Design review of the part built by this model. Coordinates are the model's own, in mm. A direction names the side the tool comes from. Round coordinates to 2 decimals unless told otherwise and drop trailing zeros. Loops run counter-clockwise (first coordinate to the right, second up) from the corner with the lowest first, then second, coordinate; pieces in that order, holes last. Notation, with made-up numbers: M 77.5,72.5 L 136.5,72.5 A14 cw 136.5,76.5 Z; hole C 24.25,-39 d7. An arc over 180 degrees is marked long. Answer as CSV lines item,"result". Start each with the question number.
from build123d import *

# Parameters (mm, degrees)
SKETCH5_W           = 1600
SKETCH5_H           = 900
BOSS_EXTRUDE4_DEPTH = 100
SKETCH6_R           = 50
BOSS_EXTRUDE5_DEPTH = 700
SKETCH8_R           = 75
CUT_EXTRUDE2_DEPTH  = 90
FILLET2_R           = 80


with BuildPart() as part:
    # Sketch5 → Boss-Extrude4 (new body)
    with BuildSketch(Plane(origin=(0, 0, 0), x_dir=(1, 0, 0), z_dir=(0, 1, 0))):
        Rectangle(SKETCH5_W, SKETCH5_H)
    extrude(amount=BOSS_EXTRUDE4_DEPTH)

    # Sketch6 → Boss-Extrude5 (add)
    with BuildSketch(Plane(origin=(0, 100, 0), x_dir=(1, 0, 0), z_dir=(0, 1, 0))):
        with Locations((-710, 360)):
            Circle(SKETCH6_R)
        with Locations((710, 360)):
            Circle(SKETCH6_R)
        with Locations((710, -360)):
            Circle(SKETCH6_R)
        with Locations((-710, -360)):
            Circle(SKETCH6_R)
    extrude(amount=-BOSS_EXTRUDE5_DEPTH)

    # Sketch8 → Cut-Extrude2 (cut)
    with BuildSketch(Plane(origin=(0, 100, 0), x_dir=(1, 0, 0), z_dir=(0, 1, 0))):
        with Locations((400, 0)):
            Circle(SKETCH8_R)
    cut_extrude2 = extrude(amount=-CUT_EXTRUDE2_DEPTH, mode=Mode.SUBTRACT)

    # Mirror1: Cut-Extrude2 across plane
    add(cut_extrude2.mirror(Plane(origin=(0, 0, 0), x_dir=(0, 0, 1), z_dir=(1, 0, 0))), mode=Mode.SUBTRACT)

    # Fillet2
    fillet2_edges = [part.edges().sort_by_distance(p)[0] for p in [
        (800, 50, 450),
        (-800, 50, 450),
        (-800, 50, -450),
        (800, 50, -450),
    ]]
    fillet(fillet2_edges, radius=FILLET2_R)


solid = part.part
Item 1: Consider section A-A, the plane z = 0. Write out the cut boundary in (x, y), then the cut area to 3 significant figures.
Item 2: Consider section B-B, the plane y = -155. Write out the cut boundary in (x, z), then the cut area to 3 significant figures.
Item 3: The part is to be moulded in two halves that separate along Z. For faces 1 (the face through (757.69, -295.8, 344.98)), 2 (the face through (-469.28, 55.63, 28.73)), 3 (the face through (775.94, 50.7, -427.19)), 4 (the face through (-777.19, 50.7, 425.94)), say which applies: +Z half, -Z half, draft (parallel to the pull), parting line (faces both ways), or undercut.
Item 4: Consider section D-D, the plane z = -138.5. Write out the cut boundary in (x, y), then the cut area to 3 significant figures.
Item 5: Insertion check: pin 1 Ø1 at (y, z) = (-244, -329.5) entering from -X; pin 2 Ø10 at (x, z) = (389, 265) entering from -Y. Each pin has a flat end and moves straight along its axis. Give the tip position at first contact, or say it passes through.
Item 6: To check wall thickness, follow line 1 (X direction, y = 56, z = 0); line 2 (Z direction, x = 400, y = 32); line 3 (Y direction, x = -663.5, z = 68.5). State the ranges of each line that lie inside material, in increasing order.
Item 7: Tool access review of faces 5 (the face through (-399, 10, -1)), 6 (the face through (757.69, -295.8, -375.02)), 7 (the face through (-777.19, 50.7, -425.94)): name each direction out of +Z, -Z, +X, -X, +Y, -Y from which nothing blocks a thin tool from reaching the whole face with its end or side.
Item 8: Consider section C-C, the plane x = -400. Write out the cut boundary in (y, z), then the cut area to 3 significant figures.
Found:
1,outline,"M -800,0 L 800,0 L 800,100 L 475,100 L 475,10 L 325,10 L 325,100 L -325,100 L -325,10 L -475,10 L -475,100 L -800,100 Z"
1,area,"133,000 mm^2"
2,outline,"C -710,-360 d100; C -710,360 d100; C 710,-360 d100; C 710,360 d100"
2,area,"31,400 mm^2"
3,face 1,"undercut"
3,face 2,"undercut"
3,face 3,"-Z half"
3,face 4,"+Z half"
4,outline,"M -800,0 L 800,0 L 800,100 L -800,100 Z"
4,area,"160,000 mm^2"
5,pin 1,"stops at x = -750"
5,pin 2,"stops at y = 0"
6,line 1,"x = -800 to -475, -325 to 325, 475 to 800"
6,line 2,"z = -450 to -75, 75 to 450"
6,line 3,"y = 0 to 100"
7,face 5,"+Y"
7,face 6,"-Y"
7,face 7,"-Z, -X, +Y, -Y"
8,outline,"M 0,-450 L 100,-450 L 100,-75 L 10,-75 L 10,75 L 100,75 L 100,450 L 0,450 Z"
8,area,"76,500 mm^2"
